Check sheet for the drawn part. Datum: minimum x, y, z corner. Units: mm. Coordinates: 2 decimals unless noted, no trailing zeros. Order: outer loops, then holes, each group sorted by start corner. A loop starts at its lowest first (then second) coordinate and runs counter-clockwise, first axis right, second up. Notation, with made-up numbers: M 44,70.5 L 95,70.5 A10 cw 95,88.5 Z; hole C 26.5,3 d11. An arc over 180 degrees is marked long. Return JSON: item names as keys, results as strings. Group by question number.
Q1. Section check D-D, the plane z = 8. Enter the section's corners in (x, y), then the cut area to 3 significant figures.
Q2. Section check C-C, the plane z = 33. Enter the section's corners in (x, y), then the cut area to 3 significant figures.
Q3. Section check B-B, the plane x = 240. Enter the section's corners in (y, z).
Q4. Go/stop test with flat-tipped pins: pin 1 Ø21 at (x, z) = (173.5, 49.5) entering from -Y; pin 2 Ø8 at (y, z) = (4, 38) entering from +X. Record where each tip stops, or that it passes through.
Q5. Section check A-A, the plane y = 14.5. Enter the section's corners in (x, z), then the cut area to 3 significant figures.
Q6. Thickness scan on probe 1 along Y at (x, z) = (49, 42); probe 2 along X at (y, z) = (4, 34.5); probe 3 along Z at (x, y) = (55.5, 22). Record the ranges inside material, lowest first.
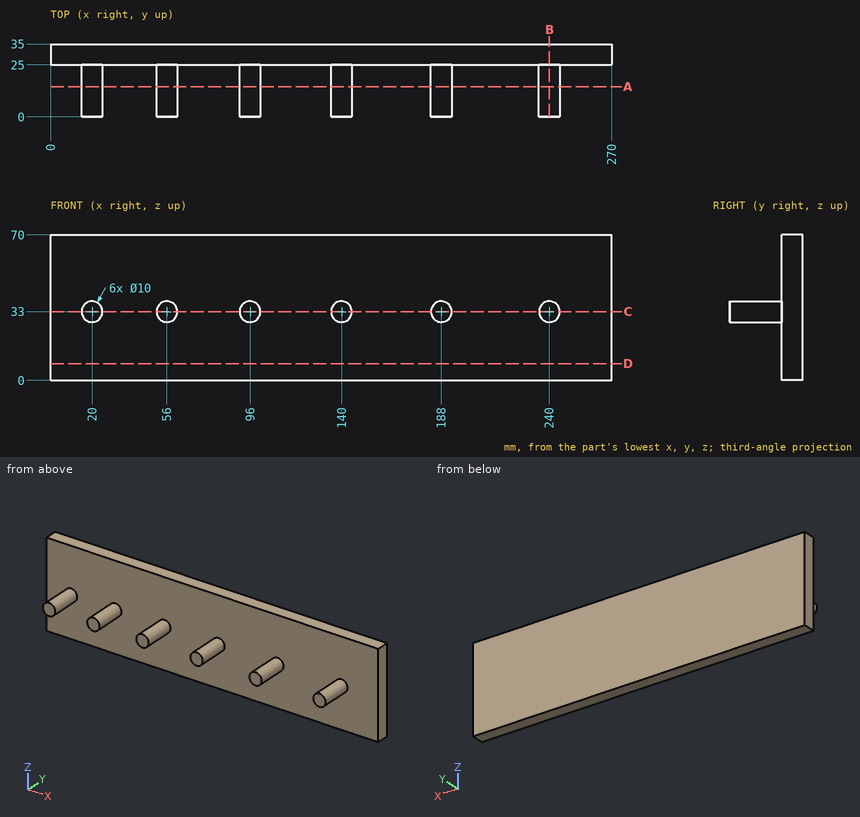
Numbers:
{
 "1": {"outline": "M 0,25 L 270,25 L 270,35 L 0,35 Z", "area": "2,700 mm2"},
 "2": {"outline": "M 0,25 L 15,25 L 15,0 L 25,0 L 25,25 L 51,25 L 51,0 L 61,0 L 61,25 L 91,25 L 91,0 L 101,0 L 101,25 L 135,25 L 135,0 L 145,0 L 145,25 L 183,25 L 183,0 L 193,0 L 193,25 L 235,25 L 235,0 L 245,0 L 245,25 L 270,25 L 270,35 L 0,35 Z", "area": "4,200 mm2"},
 "3": {"outline": "M 0,28 L 25,28 L 25,0 L 35,0 L 35,70 L 25,70 L 25,38 L 0,38 Z"},
 "4": {"pin 1": "stops at y = 25", "pin 2": "stops at x = 244.9"},
 "5": {"outline": "C 20,33 d10; C 56,33 d10; C 96,33 d10; C 140,33 d10; C 188,33 d10; C 240,33 d10", "area": "471 mm2"},
 "6": {"probe 1": "y = 25 to 35", "probe 2": "x = 15.23 to 24.77, 51.23 to 60.77, 91.23 to 100.77, 135.23 to 144.77, 183.23 to 192.77, 235.23 to 244.77", "probe 3": "z = 28.03 to 37.97"}
}
